from build123d import *

# Parameters (mm, degrees)
SKETCH1_W                    = 15
SKETCH1_H                    = 42.15
BASE_FLANGE1_DEPTH           = 3.175
EDGE_FLANGE1_STRIP_W         = 14.7
EDGE_FLANGE1_STRIP_H         = 3.175
EDGE_FLANGE1_STRIP_CUT_DEPTH = 15
EDGE_FLANGE1_DEPTH           = 15
M5_CLEARANCE_HOLE1_D         = 5.5
M4_CLEARANCE_HOLE1_D         = 4.5
FILLET1_R                    = 3.175


# Sheet-metal steps are written as plain solids
with BuildPart() as part:
    # Sketch1 → Base-Flange1 (new body)
    with BuildSketch(Plane(origin=(0, 0, 0), x_dir=(1, 0, 0), z_dir=(0, 1, 0))):
        Rectangle(SKETCH1_W, SKETCH1_H)
    extrude(amount=BASE_FLANGE1_DEPTH)

    # Edge-Flange1 strip (across the edge) → Edge-Flange1 strip cut (cut)
    with BuildSketch(Plane(origin=(7.5, 3.175, -21.075), x_dir=(0, 0, 1), z_dir=(-1, 0, 0))):
        with Locations((-3.175, -1.5875)):
            Rectangle(EDGE_FLANGE1_STRIP_W, EDGE_FLANGE1_STRIP_H)
    extrude(amount=EDGE_FLANGE1_STRIP_CUT_DEPTH, mode=Mode.SUBTRACT)

    # Edge-Flange1 section (across the edge) → Edge-Flange1 (add)
    with BuildSketch(Plane(origin=(7.5, 3.175, -21.075), x_dir=(0, 0, 1), z_dir=(-1, 0, 0))):
        with BuildLine():
            Line((0, 1), (0, 13.385))
            Line((0, 13.385), (3.175, 13.385))
            Line((3.175, 13.385), (3.175, 1))
            ThreePointArc((3.175, 1), (3.467893219, 0.292893219), (4.175, 0))
            Line((4.175, 0), (4.175, -3.175))
            ThreePointArc((4.175, -3.175), (1.222829189, -1.952170811), (0, 1))
        make_face()
    extrude(amount=EDGE_FLANGE1_DEPTH)

    # M5 Clearance Hole1 (through all)
    with Locations(Plane(origin=(0, 3.175, 0), x_dir=(1, 0, 0), z_dir=(0, 1, 0))):
        with Locations((0, -15.075)):
            Hole(M5_CLEARANCE_HOLE1_D / 2)

    # M4 Clearance Hole1 (through all)
    with Locations(Plane.XY.offset(-17.9)):
        with Locations((0, 10.56)):
            Hole(M4_CLEARANCE_HOLE1_D / 2)

    # Fillet1
    fillet1_edges = [part.edges().sort_by_distance(p)[0] for p in [
        (7.5, 16.56, -19.4875),
        (-7.5, 16.56, -19.4875),
        (7.5, 1.5875, 21.075),
        (-7.5, 1.5875, 21.075),
    ]]
    fillet(fillet1_edges, radius=FILLET1_R)


solid = part.part
Geometry: final body of the model. Coordinates: model frame, mm. A direction names the side the tool comes from. Give positions to 0.01 mm unless a question says otherwise; leave off trailing zeros. Write each loop counter-clockwise with the first axis right and the second up, starting at its lowest first coordinate (ties: lowest second). Pieces come first, ordered by that corner, then holes.
(1) Ray query, line 1 (Y direction, x = 0.5, z = 11) (3 decimals); line 2 (Z direction, x = 1.5, y = 5.25) (3 decimals); line 3 (Z direction, x = 0, y = 1.25) (3 decimals). Return the intervals inside material, ascending.
(2) Access query for faces 1 (the flat face through (0, 3.175, 2)), 2 (the cylindrical face through (-6.6, 15.6, -19.5)). Directions: +Z, -Z, +X, -X, +Y, -Y. A direction counts if a zero-diameter tool reaches every point of the face in a straight line with its end or side. Return the directions, or none.
(3) Cut plane C-C, the plane z = 15.5. Return loops of the section in (x, y) (3 decimals), then the cut area to 3 significant figures.
(4) Cut plane A-A, the plane x = 0. Return loops of the section in (y, z) (3 decimals), then the cut area to 3 significant figures.
(5) Mould query, pull axis X, two halves, no side actions, for faces 3 (the cylindrical face through (6.595, 1.61, 20.12)), 4 (the flat face through (2, 9, -17.9)), 5 (the cylindrical face through (-1.038, 8.564, -19.51)). Classes: released by +X, released by -X, zero draft, split by the parting line, or undercut.
(6) Cut plane D-D, the plane x = 5.25. Return loops of the section in (y, z) (3 decimals), then the cut area to 3 significant figures.
(7) Cut plane B-B, the plane y = 10.56. Return loops of the section in (x, z) (3 decimals), then the cut area to 3 significant figures.
Values follow:
1. line 1: y = 0 to 3.175
1. line 2: z = -21.075 to -17.9
1. line 3: z = -19.879 to 12.325, 17.825 to 21.075
2. face 1: +Z, +X, -X, +Y
2. face 2: +Z, -Z, -X, +Y
3. outline: (-7.5, 0) - (-2.717, 0) - (-2.717, 3.175) - (-7.5, 3.175) - close; (2.717, 0) - (7.5, 0) - (7.5, 3.175) - (2.717, 3.175) - close
3. area: 30.4 mm2
4. outline: (0, -16.9) arc R4.175 ccw to (4.175, -21.075) - (8.31, -21.075) - (8.31, -17.9) - (4.175, -17.9) arc R1 cw to (3.175, -16.9) - (3.175, 12.325) - (0, 12.325) - close; (0, 17.825) - (3.175, 17.825) - (3.175, 21.075) - (0, 21.075) - close; (12.81, -21.075) - (16.56, -21.075) - (16.56, -17.9) - (12.81, -17.9) - close
4. area: 141 mm2
5. face 3: released by +X
5. face 4: zero draft
5. face 5: undercut
6. outline: (0, -16.9) arc R4.175 ccw to (4.175, -21.075) - (16.422, -21.075) - (16.422, -17.9) - (4.175, -17.9) arc R1 cw to (3.175, -16.9) - (3.175, 20.937) - (0, 20.937) - close
6. area: 172 mm2
7. outline: (-7.5, -21.075) - (-2.25, -21.075) - (-2.25, -17.9) - (-7.5, -17.9) - close; (2.25, -21.075) - (7.5, -21.075) - (7.5, -17.9) - (2.25, -17.9) - close
7. area: 33.3 mm2
